Print and shaded views of the part. All mm, measured from the part's lowest x, y and z. Coordinates: 2 decimals unless noted, no trailing zeros. Loops run counter-clockwise (first coordinate to the right, second up) from the corner with the lowest first, then second, coordinate; pieces in that order, holes last.
1) Pin check, flat tip, straight feed: pin 1 Ø2 at (x, z) = (14, 4) entering from +Y. Stop position of the tip, or through.
2) Saw through at B-B, the plane y = 3.5. Write the cut outline in (x, z), and give its area (3 significant figures).
3) Saw through at A-A, the plane x = 9.5. Write the cut outline in (y, z).
4) Saw through at C-C, the plane z = 3.95. Write the cut outline in (x, y).
5) Wall check: line 1 along Z through (x, y) = (26, 2.3); line 2 along Y through (x, z) = (23, 2); line 3 along Y through (x, z) = (32, 2.9). Give the ranges that are in metal, low to high.
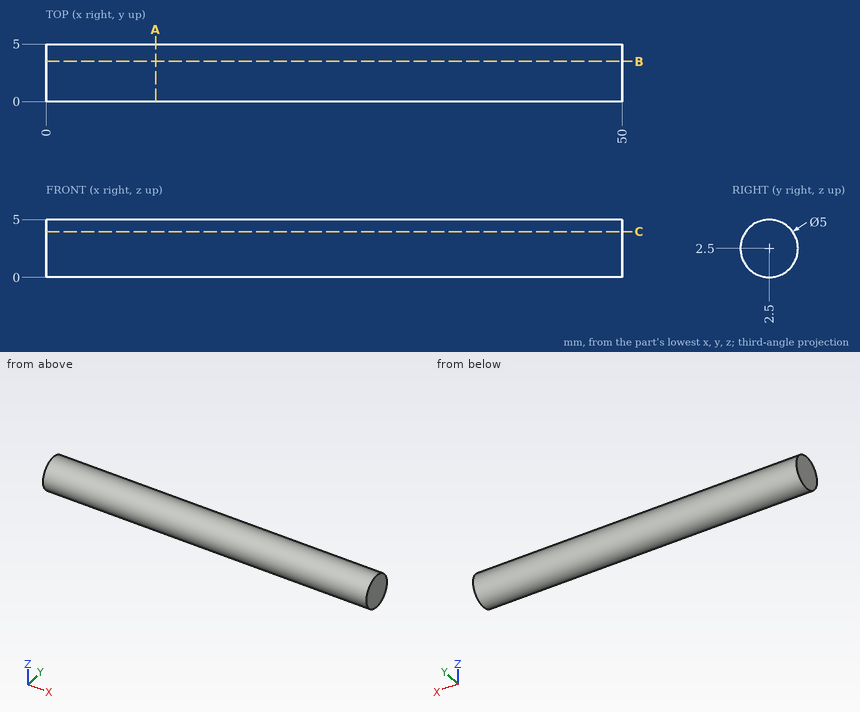
Data:
1. pin 1: stops at y = 4.95
2. outline: (0, 0.21) - (50, 0.21) - (50, 4.79) - (0, 4.79) - close
2. area: 229 mm2
3. outline: circle Ø5 at (2.5, 2.5)
4. outline: (0, 0.46) - (50, 0.46) - (50, 4.54) - (0, 4.54) - close
5. line 1: z = 0.01 to 4.99
5. line 2: y = 0.05 to 4.95
5. line 3: y = 0.03 to 4.97
